```python
from build123d import *

# Parameters (mm, degrees)
CUT_EXTRUDE_THIN2_DEPTH      = 20.052558883
CUT_EXTRUDE_THIN2_DEPTH_BACK = 1
SKETCH2_W                    = 2
SKETCH2_H                    = 26


with BuildPart() as part:
    # Sketch1 → Revolve1 (revolve)
    with BuildSketch(Plane(origin=(0, 0, 0), x_dir=(0, 0, -1), z_dir=(1, 0, 0))):
        Polygon((-13, 1.761213565), (-5.619361604, -2.5), (-4, -2.5), (-4, 2.5), (-13, 2.5), align=None)
    revolve(axis=Axis((0, 36.09806212, 0), (0, -1, 0)))

    # Sketch2 → Cut-Extrude-Thin2 (cut, two sides: drawn at the far end of the back side and taken through both)
    with BuildSketch(Plane(origin=(0, 2.5, 0), x_dir=(1, 0, 0), z_dir=(0, 1, 0)).offset(-CUT_EXTRUDE_THIN2_DEPTH_BACK)):
        Rectangle(SKETCH2_W, SKETCH2_H)
    extrude(amount=CUT_EXTRUDE_THIN2_DEPTH + CUT_EXTRUDE_THIN2_DEPTH_BACK, mode=Mode.SUBTRACT)


solid = part.part
```
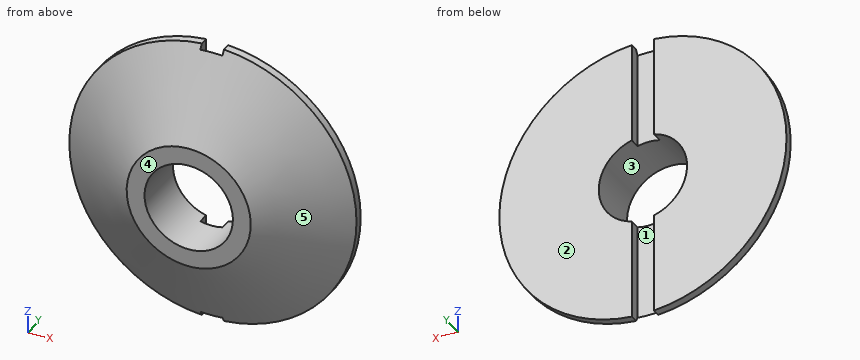
Input: part model. Units: mm. Frame: model coordinates. Face numbers are marked on the shaded views. A direction names the side the tool comes from. Round coordinates to 2 decimals unless told otherwise and drop trailing zeros. Write each loop counter-clockwise with the first axis right and the second up, starting at its lowest first coordinate (ties: lowest second). Pieces come first, ordered by that corner, then holes. Notation, with made-up numbers: (30, 71.25) -> (66, 71.25) arc R23 ccw to (66, 91.25) -> close; hole circle Ø11 at (-32, -28). An arc over 180 degrees is marked (long way). Answer as CSV lines item,"result".
1. Section B-B (z = 0). Return the cut outline in (x, y), plus the area to 3 significant figures.
Geometry says:
outline,"(-13, 1.76) -> (-5.62, -2.5) -> (-4, -2.5) -> (-4, 2.5) -> (-13, 2.5) -> close; (4, -2.5) -> (5.62, -2.5) -> (13, 1.76) -> (13, 2.5) -> (4, 2.5) -> close"
area,"58.5 mm^2"
2. Section A-A (x = 0). Return the cut outline in (y, z).
Geometry says:
outline,"(-2.5, -5.62) -> (1.5, -12.55) -> (1.5, -4) -> (-2.5, -4) -> close; (-2.5, 4) -> (1.5, 4) -> (1.5, 12.55) -> (-2.5, 5.62) -> close"
3. Reachability of the marked faces 1 and 2 from +Z, -Z, +X, -X, +Y, -Y: full face, straight path, thin tool, end or side. Return the list, or none.
Geometry says:
face 1,"+Z, -Z, +Y"
face 2,"+Z, -Z, +X, -X, +Y"
4. Mould query, pull axis X, two halves, no side actions, for the marked faces 3, 4 and 5. Classes: +X half, -X half, draft (parallel to the pull), parting line (faces both ways), or undercut.
Geometry says:
face 3,"undercut"
face 4,"draft"
face 5,"parting line"
5. Ray query, L1, parallel to X at y = -0.65, z = -2; L2, parallel to X at y = 1.8, z = -10.25; L3, parallel to Z at x = 0, y = 0.9. Return the intervals inside material, ascending. Write a range as [from, to].
Geometry says:
L1,"x = [-8.59, -3.46], [3.46, 8.59]"
L2,"x = [-8, -1], [1, 8]"
L3,"z = [-11.51, -4], [4, 11.51]"
6. Section C-C (y = -0.05). Return the cut outline in (x, z).
Geometry says:
outline,"circle Ø19.73 at (0, 0); hole circle Ø8 at (0, 0)"
7. Section D-D (y = -1.85). Return the cut outline in (x, z), plus the area to 3 significant figures.
Geometry says:
outline,"circle Ø13.49 at (0, 0); hole circle Ø8 at (0, 0)"
area,"92.7 mm^2"
8. Contact query for flat-ended pins moving along their axis: P1, Ø0.8, axis at y = 2, z = -8, coming from the -X side; P2, Ø0.8, axis at y = 2, z = -6.5, coming from the +X side; P3, Ø1.1, axis at y = 2, z = 10.5, coming from the -X side. Output: stop coordinate, or through.
Geometry says:
P1,"stops at x = -10.55"
P2,"stops at x = 11.48"
P3,"stops at x = -8.37"
